Autodesk Fusion 360 part; units mm, degrees
sketch "Sketch1" plane through (0, 0, 0) normal (0, 1, 0) x (1, 0, 0) in component "Component'"
  circle A0 centre (0, 0) radius 20
  line L0 (0, 0) -> (0, 20)
  line L1 (-35, 0) -> (-35, 60)
  line L2 (-35, 60) -> (35, 60)
  line L3 (35, 60) -> (35, 0)
  arc A1 (-35, 0) -> (35, 0) centre (0, 0) ccw
  line L4 (0, 20) -> (0, 37.5) construction
  line L5 (25, 45) -> (-25, 45)
  line L6 (-25, 45) -> (-25, 30)
  line L7 (-25, 30) -> (25, 30)
  line L8 (25, 30) -> (25, 45)
  line L9 (25, 45) -> (-25, 30) construction
  line L10 (-25, 45) -> (25, 30) construction
  point P0 (0, 37.5)
  dimension "d1" = 40
  dimension "d2" = 70
  dimension "d4" = 70
  dimension "d5" = 17.5
  dimension "d6" = 50
  dimension "d7" = 15
sketch "Sketch2" plane through (0, 0, 0) normal (0, 1, 0) x (1, 0, 0) in component "Component'"
extrude "Extrude1" add sketch "Sketch1" along normal blind 10
component "Component" placed x (1, 0, 0) y (0, 1, 0) z (0, 0, 1) at (0, 0, 0)
component "Component'" placed x (1, 0, 0) y (0, 1, 0) z (0, 0, 1) at (0, 0, 0) in component "Component"
Geometry check sheet. Reference: the model listing, model coordinates, mm. A direction names the side the tool comes from. Coordinates: 2 decimals unless noted, no trailing zeros. Order: outer loops, then holes, each group sorted by start corner. A loop starts at its lowest first (then second) coordinate and runs counter-clockwise, first axis right, second up. Notation, with made-up numbers: M 33,55.5 L 43,55.5 A22 cw 43,68.5 Z; hole C 9,36 d1. An arc over 180 degrees is marked long. Use CSV: the item, a comma, the result in double quotes.
Item 1: Tool access check on faces 1 (the flat face through (0, 5, -30)), 2 (the flat face through (0, 0, -24)). Record the directions out of +Z, -Z, +X, -X, +Y, -Y that give a thin tool (end or side, any length) a straight path to the whole face; none if there is none.
Returned:
face 1,"+Y, -Y"
face 2,"+Z, -Z, +X, -X, -Y"
Item 2: Cross-section at D-D on z = 9.5. Record the cut outline in (x, y).
Returned:
outline,"M -33.69,0 L -17.6,0 L -17.6,10 L -33.69,10 Z; M 17.6,0 L 33.69,0 L 33.69,10 L 17.6,10 Z"
Item 3: Mould release check, pull along X, two halves, no side actions. Record for faces 3 (the flat face through (0, 5, -60)), 4 (the flat face through (-25, 5, -38)), 5 (the flat face through (-35, 5, -30)): pulls with the +X half, pulls with the -X half, needs draft (parallel to the pull), parting line crosses it, or undercut.
Returned:
face 3,"needs draft"
face 4,"undercut"
face 5,"pulls with the -X half"
Item 4: Gauge pin test, flat ends, axial feed: pin 1 Ø2 at (x, y) = (-11.5, 1.5) entering from +Z; pin 2 Ø6 at (x, y) = (-13, 1.5) entering from +Z; pin 3 Ø3 at (x, z) = (12.5, 21) entering from -Y; pin 4 Ø3 at (x, z) = (6, -17) entering from -Y. Record the tip position at first contact, or that the pin passes through.
Returned:
pin 1,"stops at z = 33.39"
pin 2,"stops at z = 33.54"
pin 3,"stops at y = 0"
pin 4,"passes through"
Item 5: Cross-section at B-B on y = 5.5. Record the cut outline in (x, z), then the cut area to 3 significant figures.
Returned:
outline,"M -35,-60 L 35,-60 L 35,0 A35 ccw -35,0 Z; hole M -25,-45 L 25,-45 L 25,-30 L -25,-30 Z; hole C 0,0 d40"
area,"4,120 mm2"
Item 6: Cross-section at A-A on x = 0. Record the cut outline in (y, z), then the cut area to 3 significant figures.
Returned:
outline,"M 0,-60 L 10,-60 L 10,-45 L 0,-45 Z; M 0,-30 L 10,-30 L 10,-20 L 0,-20 Z; M 0,20 L 10,20 L 10,35 L 0,35 Z"
area,"400 mm2"
Item 7: Cross-section at C-C on z = -32.5. Record the cut outline in (x, y), then the cut area to 3 significant figures.
Returned:
outline,"M -35,0 L -25,0 L -25,10 L -35,10 Z; M 25,0 L 35,0 L 35,10 L 25,10 Z"
area,"200 mm2"
Item 8: Thickness scan on line 1 along Z through (x, y) = (0, 7); line 2 along Z through (x, y) = (-9, 2.5); line 3 along X through (y, z) = (6.25, -34). Record the ranges inside material, lowest first.
Returned:
line 1,"z = -60 to -45, -30 to -20, 20 to 35"
line 2,"z = -60 to -45, -30 to -17.86, 17.86 to 33.82"
line 3,"x = -35 to -25, 25 to 35"
